Build history of the part. All positions in model axes, mm. Round coordinates to 2 decimals unless told otherwise and drop trailing zeros. Write each loop counter-clockwise with the first axis right and the second up, starting at its lowest first coordinate (ties: lowest second). Pieces come first, ordered by that corner, then holes. Notation, with made-up numbers: (36.25, -5) - (77.25, -5) arc R19 cw to (77.25, 4) - close; hole circle Ø1 at (72, 88.25). An arc over 180 degrees is marked (long way). Answer as a JSON object with one key per item and string values. Group by question number.
Item 1: Probe line 1 (X direction, y = -20, z = 4.5); line 2 (Y direction, x = -40, z = 5.25); line 3 (X direction, y = -9.5, z = 1). List the from-to ranges inside material, lowest first. Write a range as from..to.
Item 2: Slice it at C-C, the plane x = -40.5. List the corners of the cut face in (y, z), then the cut area to 3 significant figures.
Item 3: Slice it at A-A, the plane z = 1. List the corners of the cut face in (x, y), then the cut area to 4 significant figures.
Item 4: Flat gauge pins, fed straight in: pin 1 (10 mm diameter, centred on x = -24, y = -19.5, fed in from -Z); pin 2 (4 mm diameter, centred on y = -27.5, z = 3.5, fed in from +X). Where does each tip first touch, or does it go through?
Item 5: Slice it at D-D, the plane z = 4.75. List the corners of the cut face in (x, y), then the cut area to 4 significant figures.
Item 6: Slice it at B-B, the plane y = -18.5. List the corners of the cut face in (x, z).
from build123d import *

# Parameters (mm, degrees)
EXTRUDE_2_DEPTH        = 8
HOLE_WIZARD_M3_2_D     = 2.5
HOLE_WIZARD_M3_2_DEPTH = 5


with BuildPart() as part:
    # 草图1 → 凸台-拉伸2 (new body)
    with BuildSketch(Plane.XY):
        Polygon((-42.3029947, -7.235847593), (-42.3029947, -32.235847593), (-17.3029947, -32.235847593), align=None)
    extrude(amount=EXTRUDE_2_DEPTH)

    # M3 螺纹孔2
    with Locations(Plane(origin=(-24.769421146, -24.769421146, 0), x_dir=(0.7071067811865439, -0.7071067811865511, 0), z_dir=(0.7071067811865511, 0.7071067811865439, 0))):
        with Locations((0.203782484, -4)):
            Hole(HOLE_WIZARD_M3_2_D / 2, depth=HOLE_WIZARD_M3_2_DEPTH)


solid = part.part
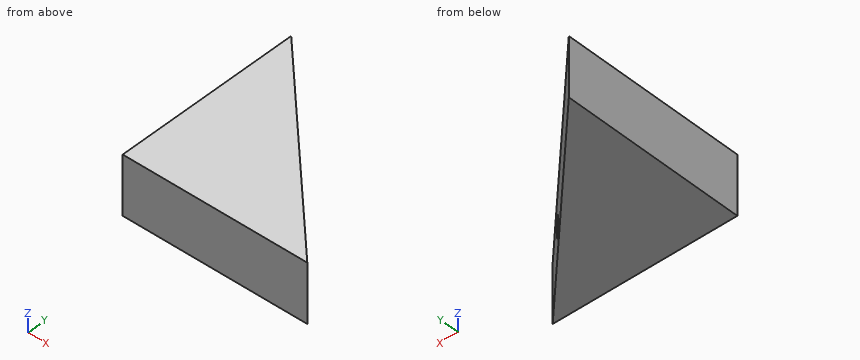
Geometry says:
{
 "1": {"line 1": "x = -42.3..-29.54", "line 2": "y = -32.24..-9.54", "line 3": "x = -42.3..-40.04"},
 "2": {"outline": "(-32.24, 0) - (-9.04, 0) - (-9.04, 8) - (-32.24, 8) - close", "area": "186 mm^2"},
 "3": {"outline": "(-42.3, -32.24) - (-17.3, -32.24) - (-42.3, -7.24) - close", "area": "312.5 mm^2"},
 "4": {"pin 1": "stops at z = 0", "pin 2": "stops at x = -20.04"},
 "5": {"outline": "(-42.3, -32.24) - (-17.3, -32.24) - (-23.92, -25.62) - (-27.45, -29.16) - (-28.87, -27.74) - (-25.33, -24.21) - (-42.3, -7.24) - close", "area": "302.5 mm^2"},
 "6": {"outline": "(-42.3, 0) - (-31.04, 0) - (-31.04, 8) - (-42.3, 8) - close"}
}
